Can you work these out from the model? Positions are in its coordinate system, mm. Give positions to 0.01 mm unless a question says otherwise; leave off trailing zeros. Order: outer loops, then holes, each group sorted by start corner. A loop starts at its lowest first (then second) coordinate and runs counter-clockwise, first axis right, second up. Notation, with made-up numbers: M 10,7.25 L 49,7.25 A26 ccw 49,25.25 Z; hole C 26,-10 d2. An arc over 180 degrees is marked long. One line per question, with ' | ' between items. Start each with the question number.
1) If we section it at D-D, the plane z = -121: Please give me the cut outline in (x, y).
2) If we section it at B-B, the plane x = 160: Please give me the cut outline in (y, z) (3 decimals), plus the area to 3 significant figures.
3) If we section it at A-A, the plane z = -134: Please give me the cut outline in (x, y), plus the area to 3 significant figures.
4) If we section it at C-C, the plane y = 67: Please give me the cut outline in (x, z).
5) Please list where these lines run through material, in increasing order: line 1 along Y through (x, z) = (134, -133.5); line 2 along Y through (x, z) = (67, -106); line 3 along Z through (x, y) = (62, 4). Write a range as [from, to].
6) I'm going to push flat-ended pins straight in: pin 1 Ø1.5 at (x, z) = (148.5, -108.5) entering from -Y; pin 2 Ø3 at (x, y) = (59.5, 12.5) entering from -Z; pin 3 Ø10 at (x, z) = (35.5, -98.5) entering from +Y; pin 4 Ø3 at (y, z) = (60.5, -115) entering from +X. Where does each tip first touch, or does it pass through?
```python
from build123d import *

# Parameters (mm, degrees)
SKETCH1_R           = 3.225
BOSS_EXTRUDE1_DEPTH = 180


with BuildPart() as part:
    # Sketch1 → Boss-Extrude1 (new body)
    with BuildSketch(Plane(origin=(0, 0, 0), x_dir=(0, 0, -1), z_dir=(1, 0, 0))):
        with BuildLine():
            Line((91.08739178, 86.768237615), (93.983652249, 89.527164089))
            ThreePointArc((93.983652249, 89.527164089), (118.199696764, 53.636477187), (129.264525293, 11.778051656))
            ThreePointArc((129.264525293, 11.778051656), (140.662275505, 4.728846729), (129.616513334, -2.860035801))
            Line((129.616513334, -2.860035801), (125.762921617, -3.054103199))
            ThreePointArc((125.762921617, -3.054103199), (117.358543926, 45.305763073), (91.08739178, 86.768237615))
        make_face()
        with Locations((132.664587351, 4.536533997)):
            Circle(SKETCH1_R, mode=Mode.SUBTRACT)
    extrude(amount=BOSS_EXTRUDE1_DEPTH)


solid = part.part
```
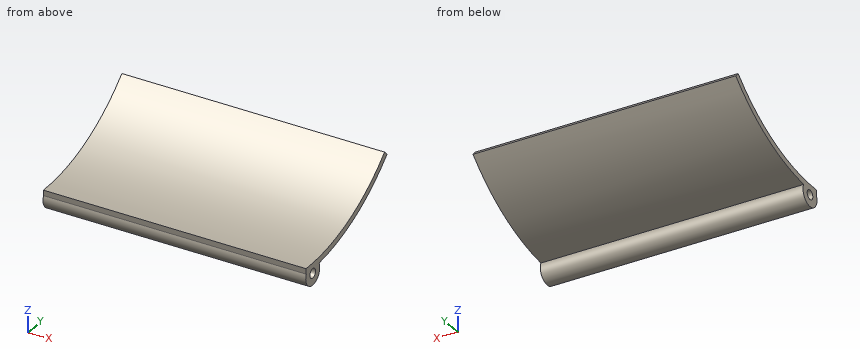
Results found:
1) outline: M 0,34.42 L 180,34.42 L 180,46.98 L 0,46.98 Z
2) outline: M -3.054,-125.763 L -2.86,-129.617 A8 ccw long 11.778,-129.265 A129.8 ccw 89.527,-93.984 L 86.768,-91.087 A125.8 cw Z; hole C 4.537,-132.665 d6.45 | area: 516 mm²
3) outline: M 0,-3.35 L 180,-3.35 L 180,1.6 L 0,1.6 Z; M 0,7.47 L 180,7.47 L 180,12.42 L 0,12.42 Z | area: 1,780 mm²
4) outline: M 0,-111.17 L 180,-111.17 L 180,-106.47 L 0,-106.47 Z
5) line 1: y = [-3.42, 1.42], [7.65, 12.49] | line 2: y = [67.75, 74.91] | line 3: z = [-140.65, -135.84], [-129.48, -125.74]
6) pin 1: stops at y = 62.37 | pin 2: stops at z = -137.38 | pin 3: stops at y = 89.53 | pin 4: stops at x = 180
